Can you work these out from the model? Positions are in its coordinate system, mm. A direction names the side the tool comes from. Give positions to 0.01 mm unless a question says otherwise; leave off trailing zeros. Loops run counter-clockwise (first coordinate to the right, second up) from the corner with the lowest first, then second, coordinate; pieces in that order, holes last. Notation, with made-up numbers: M 60.5,30 L 66.5,30 A20 ccw 66.5,62 Z; hole C 33,47 d11. An arc over 180 degrees is marked long. Use CSV: the item, a comma, the result in double quotes.
from build123d import *

# Parameters (mm, degrees)
F0_W     = 125
F0_H     = 56
F1_DEPTH = 44
F3_W     = 55
F3_H     = 12
F4_DEPTH = 13
F2_W     = 89
F2_H     = 22
F5_DEPTH = 17
F6_W     = 119
F6_H     = 38
F7_DEPTH = 52


with BuildPart() as f1:
    # F0 (on Top) → F1 (new body)
    with BuildSketch(Plane.XY):
        Rectangle(F0_W, F0_H)
    extrude(amount=-F1_DEPTH)

    # F3 (on face) → F4 (cut)
    with BuildSketch(Plane(origin=(0, 0, -44), x_dir=(1, 0, 0), z_dir=(0, 0, -1))):
        with Locations((0, -15)):
            Rectangle(F3_W, F3_H)
    extrude(amount=-F4_DEPTH, mode=Mode.SUBTRACT)

    # F2 (on face) → F5 (cut)
    with BuildSketch(Plane.XY):
        Rectangle(F2_W, F2_H)
    extrude(amount=-F5_DEPTH, mode=Mode.SUBTRACT)

    # F6 (on face) → F7 (cut)
    with BuildSketch(Plane(origin=(0, 28, 0), x_dir=(-1, 0, 0), z_dir=(0, 1, 0))):
        with Locations((0, -22)):
            Rectangle(F6_W, F6_H)
    extrude(amount=-F7_DEPTH, mode=Mode.SUBTRACT)


solid = f1.part
Q1. I want a section at D-D, the plane x = -13. Please give me the cut outline in (y, z).
Model answer:
outline,"M -28,-44 L 9,-44 L 9,-41 L -24,-41 L -24,-3 L -11,-3 L -11,0 L -28,0 Z; M 11,-3 L 28,-3 L 28,0 L 11,0 Z; M 21,-44 L 28,-44 L 28,-41 L 21,-41 Z"
Q2. Please list where these lines run through material, in increasing order: L1, parallel to X at y = 24.5, z = -34.5; L2, parallel to Z at x = 13.5, y = -12; L3, parallel to Y at x = 22, z = -25. Write a range as from..to.
Model answer:
L1,"-62.5..-59.5, 59.5..62.5"
L2,"-44..-41, -3..0"
L3,"-28..-24"
Q3. I want a section at A-A, the plane x = -42.5. Please give me the cut outline in (y, z), then the cut area to 3 significant figures.
Model answer:
outline,"M -28,-44 L 28,-44 L 28,-41 L -24,-41 L -24,-3 L -11,-3 L -11,0 L -28,0 Z; M 11,-3 L 28,-3 L 28,0 L 11,0 Z"
area,"422 mm2"
Q4. If we mould it in two halves opening along Y, with no side actions, what happens to faces 5 (the flat face through (-1, -28, -22)), 6 (the flat face through (-1, 0, -44)), 7 (the flat face through (0, 21, -43)), 8 (the flat face through (-4.9, 28, -41.5))? For each: released by +Y, released by -Y, zero draft, split by the parting line, or undercut.
Model answer:
face 5,"released by -Y"
face 6,"zero draft"
face 7,"undercut"
face 8,"released by +Y"
Q5. I want a section at B-B, the plane y = -21. Please give me the cut outline in (x, z), then the cut area to 3 significant figures.
Model answer:
outline,"M -62.5,-44 L 62.5,-44 L 62.5,0 L -62.5,0 Z; hole M -59.5,-41 L 59.5,-41 L 59.5,-3 L -59.5,-3 Z"
area,"978 mm2"
Q6. I want a section at C-C, the plane z = -10.5. Please give me the cut outline in (x, y), then the cut area to 3 significant figures.
Model answer:
outline,"M -62.5,-28 L 62.5,-28 L 62.5,28 L 59.5,28 L 59.5,-24 L -59.5,-24 L -59.5,28 L -62.5,28 Z"
area,"812 mm2"
Q7. For faces 1 (the flat face through (1, 2, -41)), 2 (the flat face through (0, 9, -43)), 3 (the flat face through (-27.5, 15, -43)), 4 (the flat face through (-1, -11, -1)), which set-ups out of +Z, -Z, +X, -X, +Y, -Y let a thin tool reach every point of the face, with its end or its side?
Model answer:
face 1,"+Y"
face 2,"+Z, -Z"
face 3,"-Z"
face 4,"+Z"
Q8. I'm going to push flat-ended pins straight in: P1, Ø10, axis at x = -17, z = -11.5, coming from the +Y side; P2, Ø3, axis at x = -1, y = -12.5, coming from the +Z side. Where does each tip first touch, or does it pass through?
Model answer:
P1,"y = -24"
P2,"z = 0"
